The model under review builds one solid part; all positions refer to its coordinate system, in mm. A direction names the side the tool comes from. Round coordinates to 2 decimals unless told otherwise and drop trailing zeros. Order: outer loops, then holes, each group sorted by start corner. A loop starts at its lowest first (then second) coordinate and runs counter-clockwise, first axis right, second up. Notation, with made-up numbers: M 78.25,6.25 L 87.25,6.25 A33 ccw 87.25,42.25 Z; hole C -25.75,57 d7. An arc over 180 degrees is marked long. Answer as a JSON object with one key per item and string values. Group by question number.
1. Add section D-D on z = 0.95. State the section outline as (x, y) points, and give its area (3 significant figures).
2. Add section A-A on z = 0. State the section outline as (x, y) points, and give its area (3 significant figures).
3. Mouldability with a two-part tool opening along Z and no side actions: class faces 1 (the face through (-6.92, -0.01, 0.12)), 2 (the face through (8.084, -0.008, -0.02)), 3 (the face through (0, 0, -0.794)), 4 (the face through (7.663, -0.008, 0.122)) as released by +Z, released by -Z, zero draft, split by the parting line, or undercut.
4. Clearance check with a flat-ended pin moving along its axis: P1, Ø0.6, axis at x = 0.5, y = 0, coming from the -Z side. State where the tip first meets the part, or that it passes through.
5. Add section B-B on x = 0. State the section outline as (y, z) points.
6. Machinability: for faces 5 (the face through (4, 0, 0.794)), 6 (the face through (-8.117, -0.008, 0.021)), which of the approach directions +Z, -Z, +X, -X, +Y, -Y give a long, thin tool a straight path to every point of the face, cutting with its end or side? Answer none if there is none.
7. Add section C-C on y = 0.35. State the section outline as (x, z) points.
8. To check wall thickness, follow probe 1 along X at (y, z) = (0.25, -0.2); probe 2 along Z at (x, y) = (0, 0.1); probe 3 along Z at (x, y) = (-1.5, -0.15). State the ranges of each line that lie inside material, in increasing order. Write a range as [from, to].
```python
from build123d import *

# Parameters (mm, degrees)
F1_DEPTH = 0.5715
F2_R     = 0.400182
F2_R_2   = 0.323313
F2_R_3   = 0.40778
F3_DEPTH = 25.4


with BuildPart() as f1:
    # F0 (on Front) → F1 (new body, symmetric)
    with BuildSketch(Plane.XZ):
        Polygon((-7.112, 0.79375), (-7.112, -0.79375), (7.112, -0.79375), (7.112, 0.79375), (0.60626, 0.79375), (-0.60626, 0.79375), align=None)
        with BuildLine():
            ThreePointArc((-7.112, 0.79375), (-8.11707, 0), (-7.112, -0.79375))
            Line((-7.112, -0.79375), (-7.112, 0.79375))
        make_face()
        with BuildLine():
            Line((7.112, 0.79375), (7.112, -0.79375))
            ThreePointArc((7.112, -0.79375), (8.084401, 0), (7.112, 0.79375))
        make_face()
        with BuildLine():
            ThreePointArc((0.60626, 0.79375), (0, 1.40001), (-0.60626, 0.79375))
            Line((-0.60626, 0.79375), (0.60626, 0.79375))
        make_face()
    extrude(amount=F1_DEPTH, both=True)

    # F2 (on face) → F3 (cut)
    with BuildSketch(Plane.XZ.offset(0.5715)):
        with Locations((-7.301104, 0)):
            Circle(F2_R)
        with Locations((0, 0.79375)):
            Circle(F2_R_2)
        with Locations((7.27424, 0)):
            Circle(F2_R_3)
    extrude(amount=-F3_DEPTH, mode=Mode.SUBTRACT)


solid = f1.part
```
Recorded:
{
 "1": {"outline": "M -0.59,-0.57 L -0.28,-0.57 L -0.28,0.57 L -0.59,0.57 Z; M 0.28,-0.57 L 0.59,-0.57 L 0.59,0.57 L 0.28,0.57 Z", "area": "0.692 mm²"},
 "2": {"outline": "M -8.12,-0.57 L -7.7,-0.57 L -7.7,0.57 L -8.12,0.57 Z; M -6.9,-0.57 L 6.87,-0.57 L 6.87,0.57 L -6.9,0.57 Z; M 7.68,-0.57 L 8.08,-0.57 L 8.08,0.57 L 7.68,0.57 Z", "area": "16.7 mm²"},
 "3": {"face 1": "undercut", "face 2": "split by the parting line", "face 3": "released by -Z", "face 4": "undercut"},
 "4": {"P1": "stops at z = -0.79"},
 "5": {"outline": "M -0.57,-0.79 L 0.57,-0.79 L 0.57,0.47 L -0.57,0.47 Z; M -0.57,1.12 L 0.57,1.12 L 0.57,1.4 L -0.57,1.4 Z"},
 "6": {"face 5": "+Z, +Y, -Y", "face 6": "+Y, -Y"},
 "7": {"outline": "M -7.11,-0.79 L 7.11,-0.79 A0.81 ccw long 7.11,0.79 L 0.61,0.79 A0.61 ccw -0.61,0.79 L -7.11,0.79 A0.82 ccw long Z; hole C -7.3,0 d0.8; hole C 0,0.79 d0.65; hole C 7.27,0 d0.82"},
 "8": {"probe 1": "x = [-8.09, -7.65], [-6.95, 6.92], [7.63, 8.06]", "probe 2": "z = [-0.79, 0.47], [1.12, 1.4]", "probe 3": "z = [-0.79, 0.79]"}
}
